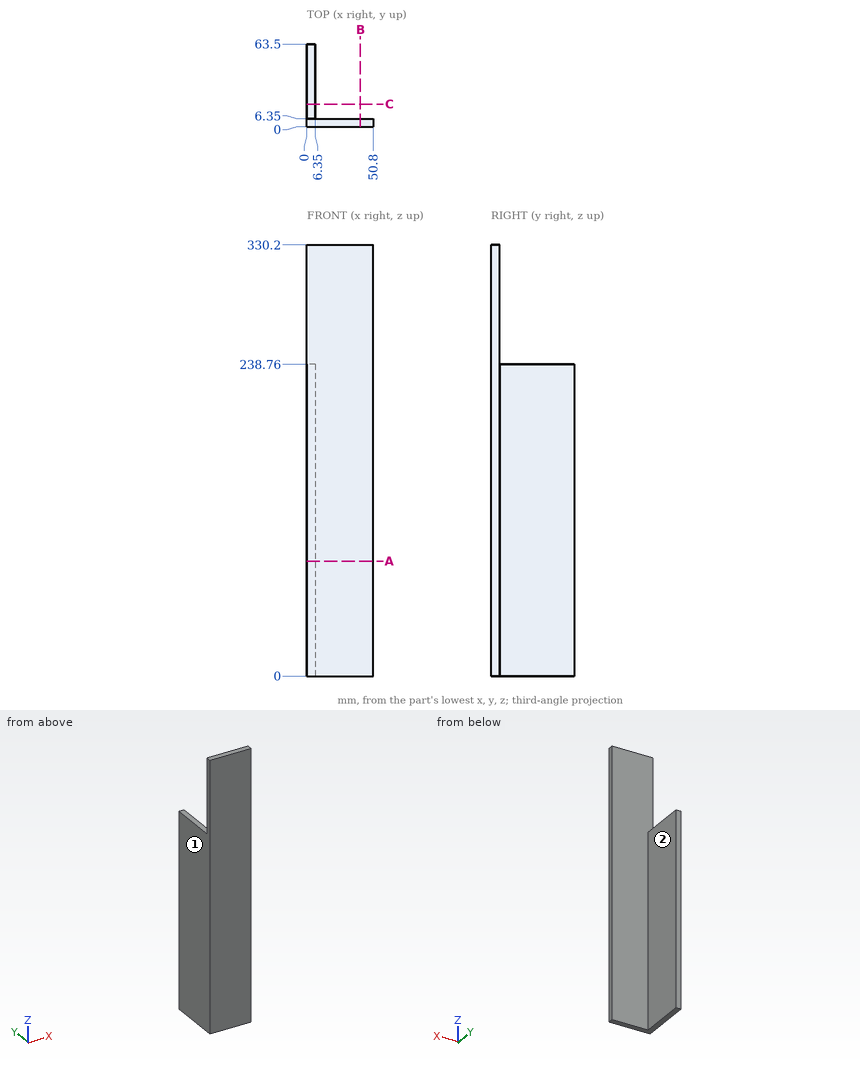
Print and shaded views of the part. All mm, measured from the part's lowest x, y and z. A direction names the side the tool comes from. Coordinates: 2 decimals unless noted, no trailing zeros. Order: outer loops, then holes, each group sorted by start corner. A loop starts at its lowest first (then second) coordinate and runs counter-clockwise, first axis right, second up. Notation, with made-up numbers: M 30.25,82 L 50.25,82 A27 cw 50.25,113 Z; hole C 20,-12 d9. An arc over 180 degrees is marked long. Write each question's results on one line, items separated by ' | '. Start each with the question number.
Q1. Drill centre lines: probe 1 along Y at (x, z) = (14, 105); probe 2 along Z at (x, y) = (4.5, 60.5). Where is each one in solid material? Low to high. Write a range as from..to.
Q2. Which spindle directions (+Z, -Z, +X, -X, +Y, -Y) get a long thin tool onto all of the face, cutting with end or side? Do the marked faces 1 and 2. Say none if no direction does.
Q3. Cut at C-C (y = 17.5). List the corners of the cut face in (x, z).
Q4. Flat gauge pins, fed straight in: P1, Ø6, axis at x = 34.5, z = 85, coming from the +Y side; P2, Ø1, axis at y = 48, z = 39.5, coming from the +X side; P3, Ø5, axis at x = 3, y = 23, coming from the +Z side; P4, Ø1, axis at x = 20.5, z = 141.5, coming from the -Y side. Where does each tip first touch, or does it go through?
Q5. Cut at B-B (x = 41). List the corners of the cut face in (y, z).
Q6. Cut at A-A (z = 88). List the corners of the cut face in (x, y), then the cut area to 3 significant figures.
Found:
1) probe 1: 0..6.35 | probe 2: 0..238.76
2) face 1: +Z, -Z, -X, +Y, -Y | face 2: +Z, -Z, +X, +Y
3) outline: M 0,0 L 6.35,0 L 6.35,238.76 L 0,238.76 Z
4) P1: y = 6.35 | P2: x = 6.35 | P3: z = 238.76 | P4: y = 0
5) outline: M 0,0 L 6.35,0 L 6.35,330.2 L 0,330.2 Z
6) outline: M 0,0 L 50.8,0 L 50.8,6.35 L 6.35,6.35 L 6.35,63.5 L 0,63.5 Z | area: 685 mm²
